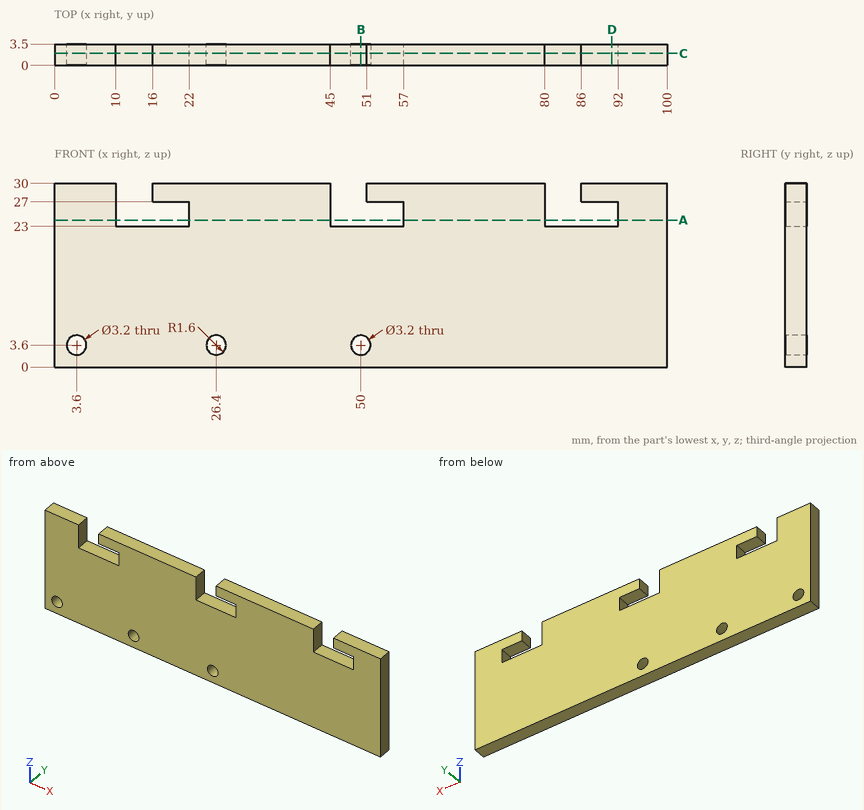
Job drawing, mm, ordinate dimensions from the low corner. One solid piece. Give positions to 0.01 mm unless a question says otherwise; leave off trailing zeros. Loops run counter-clockwise (first coordinate to the right, second up) from the corner with the lowest first, then second, coordinate; pieces in that order, holes last. Notation, with made-up numbers: (-33.5, -32) -> (-7.5, -32) arc R13 cw to (-7.5, -20) -> close; hole circle Ø8 at (2.5, -33). An arc over 180 degrees is marked (long way). Write each question's results on one line, items separated by ' | '. Start each with the question number.
Q1. Pin check, flat tips, straight feed: P1, Ø1.8, axis at x = 13.5, y = 1.5, coming from the +Z side; P2, Ø1.5, axis at y = 2, z = 29, coming from the -X side. Stop position of each tip, or through.
Q2. Band-saw the part on C-C on y = 1.95. List the corners of the cut face in (x, z), plus the area to 3 significant figures.
Q3. Band-saw the part on A-A on z = 24. List the corners of the cut face in (x, y).
Q4. Band-saw the part on D-D on x = 91. List the corners of the cut face in (y, z).
Q5. Wall check: L1, parallel to X at y = 0.45, z = 26.5; L2, parallel to Z at x = 87.5, y = 2.9; L3, parallel to Z at x = 3.6, y = 2.1. Give the ranges that are in metal, low to high.
Q6. Band-saw the part on B-B on x = 50. List the corners of the cut face in (y, z).
Results are:
1) P1: stops at z = 23 | P2: stops at x = 0
2) outline: (0, 0) -> (100, 0) -> (100, 30) -> (86, 30) -> (86, 27) -> (92, 27) -> (92, 23) -> (80, 23) -> (80, 30) -> (51, 30) -> (51, 27) -> (57, 27) -> (57, 23) -> (45, 23) -> (45, 30) -> (16, 30) -> (16, 27) -> (22, 27) -> (22, 23) -> (10, 23) -> (10, 30) -> (0, 30) -> close; hole circle Ø3.2 at (3.6, 3.6); hole circle Ø3.2 at (26.4, 3.6); hole circle Ø3.2 at (50, 3.6) | area: 2,780 mm²
3) outline: (0, 0) -> (10, 0) -> (10, 3.5) -> (0, 3.5) -> close; (22, 0) -> (45, 0) -> (45, 3.5) -> (22, 3.5) -> close; (57, 0) -> (80, 0) -> (80, 3.5) -> (57, 3.5) -> close; (92, 0) -> (100, 0) -> (100, 3.5) -> (92, 3.5) -> close
4) outline: (0, 0) -> (3.5, 0) -> (3.5, 23) -> (0, 23) -> close; (0, 27) -> (3.5, 27) -> (3.5, 30) -> (0, 30) -> close
5) L1: x = 0 to 10, 22 to 45, 57 to 80, 92 to 100 | L2: z = 0 to 23, 27 to 30 | L3: z = 0 to 2, 5.2 to 30
6) outline: (0, 0) -> (3.5, 0) -> (3.5, 2) -> (0, 2) -> close; (0, 5.2) -> (3.5, 5.2) -> (3.5, 23) -> (0, 23) -> close
